Design review of the part shown in the three views and the two pictorial views. Dimensions are in mm from the part's minimum x, y and z. Coordinates: 2 decimals unless noted, no trailing zeros. Order: outer loops, then holes, each group sorted by start corner. A loop starts at its lowest first (then second) coordinate and runs counter-clockwise, first axis right, second up. Notation, with made-up numbers: M 42.25,86 L 90.25,86 A27 ccw 90.25,114 Z; hole C 53.5,64.5 d5. An arc over 180 degrees is marked long. Use CSV: the item, a comma, the result in double quotes.
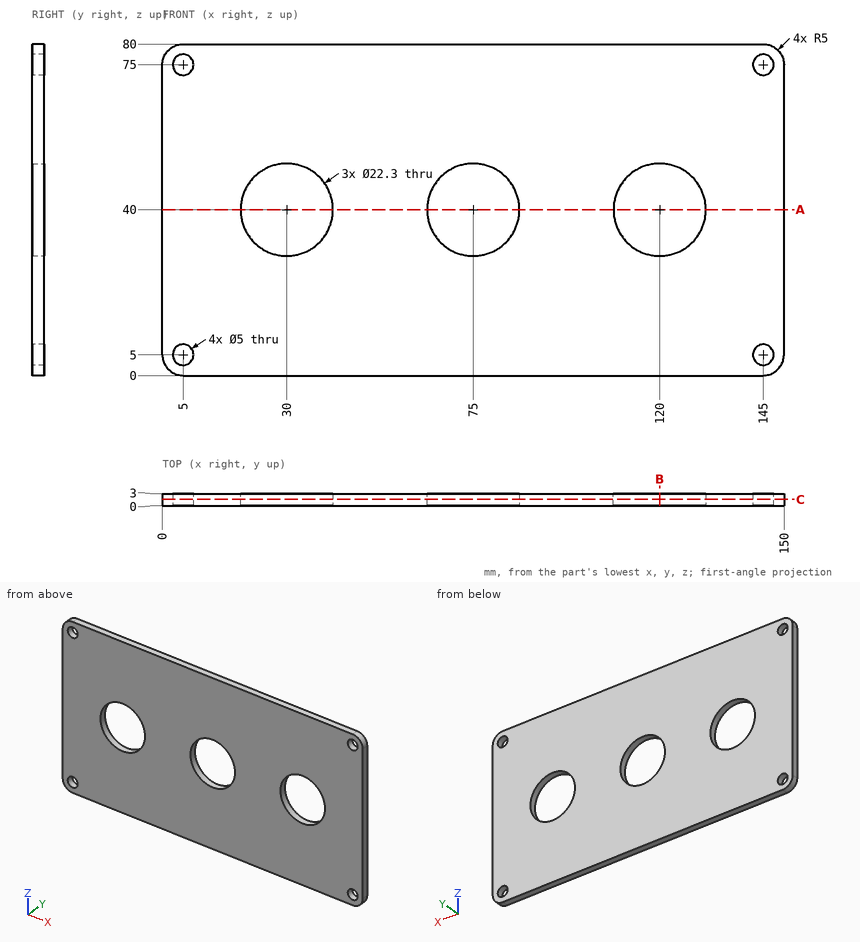
(1) Add section B-B on x = 120. State the section outline as (y, z) points.
The answers:
outline,"M 0,0 L 3,0 L 3,28.85 L 0,28.85 Z; M 0,51.15 L 3,51.15 L 3,80 L 0,80 Z"
(2) Clearance check with a flat-ended pin moving along its axis: P1, Ø6.5, axis at x = 145, z = 75, coming from the -Y side. State where the tip first meets the part, or that it passes through.
The answers:
P1,"stops at y = 0"
(3) Add section A-A on z = 40. State the section outline as (x, y) points.
The answers:
outline,"M 0,0 L 18.85,0 L 18.85,3 L 0,3 Z; M 41.15,0 L 63.85,0 L 63.85,3 L 41.15,3 Z; M 86.15,0 L 108.85,0 L 108.85,3 L 86.15,3 Z; M 131.15,0 L 150,0 L 150,3 L 131.15,3 Z"
(4) Wall thickness on probe 1 along Z at (x, y) = (145, 2.05); probe 2 along Z at (x, y) = (75, 2); probe 3 along X at (y, z) = (0.9, 34): over which ranges is each line inside the solid? List them lowest first.
The answers:
probe 1,"z = 0 to 2.5, 7.5 to 72.5, 77.5 to 80"
probe 2,"z = 0 to 28.85, 51.15 to 80"
probe 3,"x = 0 to 20.6, 39.4 to 65.6, 84.4 to 110.6, 129.4 to 150"
(5) Add section C-C on y = 1.6. State the section outline as (x, z) points.
The answers:
outline,"M 0,5 A5 ccw 5,0 L 145,0 A5 ccw 150,5 L 150,75 A5 ccw 145,80 L 5,80 A5 ccw 0,75 Z; hole C 5,5 d5; hole C 5,75 d5; hole C 30,40 d22.3; hole C 75,40 d22.3; hole C 120,40 d22.3; hole C 145,5 d5; hole C 145,75 d5"
